Geometry check sheet. Reference: the model listing, model coordinates, mm. A direction names the side the tool comes from. Coordinates: 2 decimals unless noted, no trailing zeros. Order: outer loops, then holes, each group sorted by start corner. A loop starts at its lowest first (then second) coordinate and runs counter-clockwise, first axis right, second up.
```python
from build123d import *

# Parameters (mm, degrees)
SKETCH_R        = 1
SKETCH_W        = 13.8
SKETCH_H        = 24.5
PAD_DEPTH       = 12
SKETCH001_R     = 3.5
POCKET_DEPTH    = 37.001
POCKET001_DEPTH = 3


with BuildPart() as part:
    # Sketch → Pad (new body)
    with BuildSketch(Plane.XY):
        Polygon((-30, 18.5), (10, 18.5), (10, -18.5), (-30, -18.5), (-30, -14.719735), (-10, -14.719735), (-10, 14.719735), (-30, 14.719735), align=None)
        with Locations((0, -14)):
            Circle(SKETCH_R, mode=Mode.SUBTRACT)
        with Locations((0, 14)):
            Circle(SKETCH_R, mode=Mode.SUBTRACT)
        Rectangle(SKETCH_W, SKETCH_H, mode=Mode.SUBTRACT)
    extrude(amount=PAD_DEPTH)

    # Sketch001 (on Face2 of Pad) → Pocket (cut, through all)
    with BuildSketch(Plane(origin=(0, 18.5, 0), x_dir=(-1, 0, 0), z_dir=(0, 1, 0))):
        with Locations((23.76671, 6)):
            Circle(SKETCH001_R)
    extrude(amount=-POCKET_DEPTH, mode=Mode.SUBTRACT)

    # Sketch002 → Pocket001 (cut)
    with BuildSketch(Plane.XZ.offset(-19)):
        with BuildLine():
            Line((-23.237058, 9.964646), (-8.500146, 7.979621))
            ThreePointArc((-8.505437, 4.019625), (-6.784928, 5.997328), (-8.500146, 7.979621))
            Line((-23.242355, 2.034648), (-8.505437, 4.019625))
            ThreePointArc((-23.237058, 9.964646), (-27.767697, 6.002672), (-23.242355, 2.034648))
        make_face()
    extrude(amount=POCKET001_DEPTH, mode=Mode.SUBTRACT)


solid = part.part
```
Item 1: Thickness scan on line 1 along Y through (x, z) = (0, 2.5); line 2 along X through (y, z) = (17.4, 6); line 3 along X through (y, z) = (-12, 10.25). Record the ranges inside material, lowest first.
Item 2: Release check for a two-part mould opening along Z. For faces 4 (the face through (10, 0, 6)), 5 (the face through (-9.7, 0.3, 12)), 6 (the face through (-15.977, 17.268, 3.013)) record: pulls with the +Z half, pulls with the -Z half, needs draft (parallel to the pull), parting line crosses it, or undercut.
Item 3: Sectioned sample at A-A (z = 6). Record the cut outline in (x, y).
Item 4: Depth check by flat-ended pin: P1, Ø1.5, axis at x = -20, z = 3, coming from the +Y side; P2, Ø2.5, axis at x = -20.5, z = 5.5, coming from the +Y side; P3, Ø5, axis at x = -23.77, z = 6, coming from the -Y side. Enter the tip coordinate at first touch or a pass-through.
Item 5: Sectioned sample at C-C (x = 0). Record the cut outline in (y, z), and give its area (3 significant figures).
Item 6: Sectioned sample at B-B (y = -9). Record the cut outline in (x, z), and give its area (3 significant figures).
Item 7: Sectioned sample at D-D (z = 10.75). Record the cut outline in (x, y), and give its area (3 significant figures).
Item 8: Tool access check on faces 1 (the face through (-6.9, 0, 6)), 2 (the face through (-20, -14.72, 6)), 3 (the face through (-6.785, 17.268, 5.957)). Record the directions out of +Z, -Z, +X, -X, +Y, -Y that give a thin tool (end or side, any length) a straight path to the whole face; none if there is none.
Geometry check:
1. line 1: y = -18.5 to -15, -13 to -12.25, 12.25 to 13, 15 to 18.5
1. line 2: x = -30 to -27.77, -6.78 to 10
1. line 3: x = -10 to -6.9, 6.9 to 10
2. face 4: needs draft
2. face 5: pulls with the +Z half
2. face 6: undercut
3. outline: (-30, -18.5) - (-27.27, -18.5) - (-27.27, -14.72) - (-30, -14.72) - close; (-30, 14.72) - (-27.27, 14.72) - (-27.27, 16) - (-27.77, 16) - (-27.77, 18.5) - (-30, 18.5) - close; (-20.27, -18.5) - (10, -18.5) - (10, 18.5) - (-6.78, 18.5) - (-6.78, 16) - (-20.27, 16) - (-20.27, 14.72) - (-10, 14.72) - (-10, -14.72) - (-20.27, -14.72) - close; hole (-6.9, -12.25) - (6.9, -12.25) - (6.9, 12.25) - (-6.9, 12.25) - close; hole circle Ø2 at (0, -14); hole circle Ø2 at (0, 14)
4. P1: stops at y = 18.5
4. P2: stops at y = 16
4. P3: passes through
5. outline: (-18.5, 0) - (-15, 0) - (-15, 12) - (-18.5, 12) - close; (-13, 0) - (-12.25, 0) - (-12.25, 12) - (-13, 12) - close; (12.25, 0) - (13, 0) - (13, 12) - (12.25, 12) - close; (15, 0) - (18.5, 0) - (18.5, 12) - (15, 12) - close
5. area: 102 mm2
6. outline: (-10, 0) - (-6.9, 0) - (-6.9, 12) - (-10, 12) - close; (6.9, 0) - (10, 0) - (10, 12) - (6.9, 12) - close
6. area: 74.4 mm2
7. outline: (-30, -18.5) - (10, -18.5) - (10, 18.5) - (-30, 18.5) - (-30, 14.72) - (-10, 14.72) - (-10, -14.72) - (-30, -14.72) - close; hole (-6.9, -12.25) - (6.9, -12.25) - (6.9, 12.25) - (-6.9, 12.25) - close; hole circle Ø2 at (0, -14); hole circle Ø2 at (0, 14)
7. area: 547 mm2
8. face 1: +Z, -Z
8. face 2: +Z, -Z, -X
8. face 3: +Y
